from build123d import *

# Parameters (mm, degrees)
SKETCH1_W           = 25
SKETCH1_H           = 35
BOSS_EXTRUDE1_DEPTH = 40
FILLET1_RADIUS      = 17.5
FILLET1_LENGTH      = 25
SKETCH2_W           = 15
SKETCH2_H           = 35
CUT_EXTRUDE1_DEPTH  = 30
SKETCH3_R           = 6.5
CUT_EXTRUDE2_DEPTH  = 30
SKETCH5_R           = 30
BOSS_EXTRUDE2_DEPTH = 7
SKETCH6_R           = 10
SKETCH6_R_2         = 5
BOSS_EXTRUDE3_DEPTH = 100


with BuildPart() as part:
    # Sketch1 → Boss-Extrude1 (new body)
    with BuildSketch(Plane(origin=(0, 0, 0), x_dir=(1, 0, 0), z_dir=(0, 1, 0))):
        Rectangle(SKETCH1_W, SKETCH1_H)
    extrude(amount=BOSS_EXTRUDE1_DEPTH)

    # Fillet1: full round fillet: the end face becomes a half cylinder, R = half its width
    fillet1_face = Plane((0, 0, 0), x_dir=(-1, 0, 0), z_dir=(0, -1, 0))  # on the end face: x along it, z out of the body
    fillet1_slab = fillet1_face.offset(-FILLET1_RADIUS / 2) * Box(FILLET1_LENGTH, 2 * FILLET1_RADIUS, FILLET1_RADIUS, mode=Mode.PRIVATE)  # the body's end, R deep
    fillet1_round = Plane((0, 17.5, 0), x_dir=(0, -1, 0), z_dir=(-1, 0, 0)) * Cylinder(FILLET1_RADIUS, FILLET1_LENGTH, mode=Mode.PRIVATE)  # its axis R under the face
    add(fillet1_slab - fillet1_round, mode=Mode.SUBTRACT)

    # Sketch2 → Cut-Extrude1 (cut)
    with BuildSketch(Plane(origin=(0, 0, 0), x_dir=(1, 0, 0), z_dir=(0, 1, 0))):
        Rectangle(SKETCH2_W, SKETCH2_H)
    extrude(amount=CUT_EXTRUDE1_DEPTH, mode=Mode.SUBTRACT)

    # Sketch3 → Cut-Extrude2 (cut)
    with BuildSketch(Plane.ZY.offset(12.5)):
        with Locations((0, 17.5)):
            Circle(SKETCH3_R)
    extrude(amount=-CUT_EXTRUDE2_DEPTH, mode=Mode.SUBTRACT)

    # Sketch5 → Boss-Extrude2 (add)
    with BuildSketch(Plane(origin=(0, 40, 0), x_dir=(1, 0, 0), z_dir=(0, 1, 0))):
        with Locations(Location((0, 0, 0), (0, 0, 270))):
            Circle(SKETCH5_R)
    extrude(amount=BOSS_EXTRUDE2_DEPTH)

    # Sketch6 → Boss-Extrude3 (add)
    with BuildSketch(Plane(origin=(0, 47, 0), x_dir=(1, 0, 0), z_dir=(0, 1, 0))):
        with Locations(Location((0, 0, 0), (0, 0, 270))):
            Circle(SKETCH6_R)
        with Locations(Location((0, 0, 0), (0, 0, 270))):
            Circle(SKETCH6_R_2, mode=Mode.SUBTRACT)
    extrude(amount=BOSS_EXTRUDE3_DEPTH)


solid = part.part
Design review of the part built by this model. Coordinates are the model's own, in mm. A direction names the side the tool comes from. Round coordinates to 2 decimals unless told otherwise and drop trailing zeros. Loops run counter-clockwise (first coordinate to the right, second up) from the corner with the lowest first, then second, coordinate; pieces in that order, holes last. Notation, with made-up numbers: M 76.25,64 L 98.25,64 A16 cw 98.25,88 Z; hole C 34,-10.75 d8. An arc over 180 degrees is marked long. Answer as a JSON object with one key per item and string values.
Item 1: We need section C-C on y = 21. Give the boundary of the cut face in (x, z).
Answer sheet:
{"outline": "M -12.5,-17.5 L -7.5,-17.5 L -7.5,-5.48 L -12.5,-5.48 Z; M -12.5,5.48 L -7.5,5.48 L -7.5,17.5 L -12.5,17.5 Z; M 7.5,-17.5 L 12.5,-17.5 L 12.5,-5.48 L 7.5,-5.48 Z; M 7.5,5.48 L 12.5,5.48 L 12.5,17.5 L 7.5,17.5 Z"}
Item 2: Wall thickness on L1, parallel to Z at x = 0.5, y = 63; L2, parallel to X at y = 15, z = 15.5; L3, parallel to Y at x = -9, z = 0: over which ranges is each line inside the solid? List them lowest first. Write a range as from..to.
Answer sheet:
{"L1": "z = -9.99..-4.97, 4.97..9.99", "L2": "x = -12.5..-7.5, 7.5..12.5", "L3": "y = 0..11, 24..147"}
Item 3: The part is to be moulded in two halves that separate along Z. For faces 1 (the flat face through (-13, 40, 0)), 2 (the cylindrical face through (-10.035, 23.945, -0.846)), 3 (the flat face through (0, 31, 17.5)), say which applies: pulls with the +Z half, pulls with the -Z half, needs draft (parallel to the pull), parting line crosses it, or undercut.
Answer sheet:
{"face 1": "needs draft", "face 2": "undercut", "face 3": "pulls with the +Z half"}
Item 4: Machinability: for faces 4 (the flat face through (0, 31, -17.5)), 5 (the flat face through (-12.5, 24.2, 0.2)), 6 (the flat face through (0, 47, 13)), which of the approach directions +Z, -Z, +X, -X, +Y, -Y give a long, thin tool a straight path to every point of the face, cutting with its end or side? Answer none if there is none.
Answer sheet:
{"face 4": "-Z, +X, -X, -Y", "face 5": "+Z, -Z, -X, -Y", "face 6": "+Y"}
Item 5: We need section A-A on z = 0. Give the boundary of the cut face in (x, y), and give its area (3 significant figures).
Answer sheet:
{"outline": "M -30,40 L -12.5,40 L -12.5,24 L -7.5,24 L -7.5,30 L 7.5,30 L 7.5,24 L 12.5,24 L 12.5,40 L 30,40 L 30,47 L 10,47 L 10,147 L 5,147 L 5,47 L -5,47 L -5,147 L -10,147 L -10,47 L -30,47 Z; M -12.5,0 L -7.5,0 L -7.5,11 L -12.5,11 Z; M 7.5,0 L 12.5,0 L 12.5,11 L 7.5,11 Z", "area": "1,840 mm^2"}
Item 6: Clearance check with flat-ended pins moving along their axes: P1, Ø3, axis at y = 50, z = 5, coming from the +X side; P2, Ø11.5, axis at x = 0, z = 0, coming from the -Y side; P3, Ø24, axis at y = 19.5, z = -4, coming from the +X side. State where each tip first meets the part, or that it passes through.
Answer sheet:
{"P1": "stops at x = 9.37", "P2": "stops at y = 30", "P3": "stops at x = 12.5"}
Item 7: We need section D-D on y = 114. Give the boundary of the cut face in (x, z), and give its area (3 significant figures).
Answer sheet:
{"outline": "C 0,0 d20; hole C 0,0 d10", "area": "236 mm^2"}
Item 8: We need section B-B on x = 0. Give the boundary of the cut face in (y, z).
Answer sheet:
{"outline": "M 30,-17.5 L 40,-17.5 L 40,-30 L 47,-30 L 47,-10 L 147,-10 L 147,-5 L 47,-5 L 47,5 L 147,5 L 147,10 L 47,10 L 47,30 L 40,30 L 40,17.5 L 30,17.5 Z"}
